Part model, mm, in its own coordinate system. A direction names the side the tool comes from. Round coordinates to 2 decimals unless told otherwise and drop trailing zeros. Write each loop counter-clockwise with the first axis right and the second up, starting at its lowest first coordinate (ties: lowest second). Pieces come first, ordered by that corner, then holes.
1) Which spindle directions (+Z, -Z, +X, -X, +Y, -Y) get a long thin tool onto all of the face, cutting with end or side? Do faces 4 (the flat face through (0, 48, -54)), 5 (the flat face through (-10, 63.4, -58)), 6 (the flat face through (-4, 48, -41)), 7 (the flat face through (41, 48, 4)), 8 (the cylindrical face through (63.85, 64.96, 9.86)). Say none if no direction does.
2) Flat gauge pins, fed straight in: pin 1 (8 mm diameter, centred on x = 19.5, y = 34, fed in from -Z); pin 2 (11 mm diameter, centred on y = 35.5, z = -31.5, fed in from +X); pin 3 (10.5 mm diameter, centred on y = 31.5, z = -55, fed in from +X). Where does each tip first touch, or does it go through?
3) Saw through at C-C on z = -26. Write the cut outline in (x, y).
4) Saw through at D-D on x = 39. Write the cut outline in (y, z).
5) Saw through at A-A on x = -5. Write the cut outline in (y, z).
6) Pull direction Y, two halves, no side cores. Call faces 1 (the flat face through (65.75, 48, 9)), 2 (the flat face through (58, 46.6, 10)), 3 (the cylindrical face through (52.65, 25.04, 9.86)): +Y half, -Y half, draft (parallel to the pull), parting line (faces both ways), or undercut.
7) Saw through at B-B on y = 80.5. Write the cut outline in (x, z), and give its area (3 significant figures).
8) Drill centre lines: L1, parallel to Z at x = 14, y = 57.5; L2, parallel to Z at x = -6, y = 28; L3, parallel to Z at x = 52.5, y = 51. Where is each one in solid material? Low to high.
```python
from build123d import *

# Parameters (mm, degrees)
BOSS_EXTRUDE1_DEPTH = 100
SKETCH2_W           = 37
SKETCH2_H           = 112.688383797
CUT_EXTRUDE1_DEPTH  = 7
SKETCH3_W           = 37
SKETCH3_H           = 114.700676364
CUT_EXTRUDE2_DEPTH  = 7
CUT_EXTRUDE3_DEPTH  = 148.228139294
CUT_EXTRUDE4_DEPTH  = 137.550814717
FILLET1_R           = 10
FILLET2_R           = 2
FILLET3_R           = 2
FILLET4_R           = 2


with BuildPart() as part:
    # Sketch1 → Boss-Extrude1 (new body)
    with BuildSketch(Plane(origin=(0, 0, 0), x_dir=(1, 0, 0), z_dir=(0, 1, 0))):
        Polygon((0, 0), (65.75, 0), (65.75, -20), (-20, -20), (-20, 65.75), (0, 65.75), align=None)
    extrude(amount=BOSS_EXTRUDE1_DEPTH)

    # Sketch2 → Cut-Extrude1 (cut)
    with BuildSketch(Plane(origin=(0, 0, 0), x_dir=(0, 0, -1), z_dir=(1, 0, 0))):
        with Locations((22.5, 52.54890392)):
            Rectangle(SKETCH2_W, SKETCH2_H)
    extrude(amount=-CUT_EXTRUDE1_DEPTH, mode=Mode.SUBTRACT)

    # Sketch3 → Cut-Extrude2 (cut)
    with BuildSketch(Plane(origin=(0, 0, 0), x_dir=(-1, 0, 0), z_dir=(0, 0, -1))):
        with Locations((-22.5, 48.993853716)):
            Rectangle(SKETCH3_W, SKETCH3_H)
    extrude(amount=-CUT_EXTRUDE2_DEPTH, mode=Mode.SUBTRACT)

    # Sketch4 → Cut-Extrude3 (cut, through all)
    with BuildSketch(Plane.ZY.offset(20)):
        with BuildLine():
            Line((-62.25, 86.6), (-54.25, 86.6))
            ThreePointArc((-54.25, 86.6), (-52.65, 85), (-54.25, 83.4))
            Line((-54.25, 83.4), (-62.25, 83.4))
            ThreePointArc((-62.25, 83.4), (-63.85, 85), (-62.25, 86.6))
        make_face()
        with BuildLine():
            Line((-62.25, 66.6), (-54.25, 66.6))
            ThreePointArc((-54.25, 66.6), (-52.65, 65), (-54.25, 63.4))
            Line((-54.25, 63.4), (-62.25, 63.4))
            ThreePointArc((-62.25, 63.4), (-63.85, 65), (-62.25, 66.6))
        make_face()
        with BuildLine():
            Line((-62.25, 46.6), (-54.25, 46.6))
            ThreePointArc((-54.25, 46.6), (-52.65, 45), (-54.25, 43.4))
            Line((-54.25, 43.4), (-62.25, 43.4))
            ThreePointArc((-62.25, 43.4), (-63.85, 45), (-62.25, 46.6))
        make_face()
        with BuildLine():
            Line((-62.25, 26.6), (-54.25, 26.6))
            ThreePointArc((-54.25, 26.6), (-52.65, 25), (-54.25, 23.4))
            Line((-54.25, 23.4), (-62.25, 23.4))
            ThreePointArc((-62.25, 23.4), (-63.85, 25), (-62.25, 26.6))
        make_face()
    extrude(amount=-CUT_EXTRUDE3_DEPTH, mode=Mode.SUBTRACT)

    # Sketch6 → Cut-Extrude4 (cut, through all)
    with BuildSketch(Plane(origin=(0, 0, 0), x_dir=(-1, 0, 0), z_dir=(0, 0, -1))):
        with BuildLine():
            Line((-62.25, 86.6), (-54.25, 86.6))
            ThreePointArc((-54.25, 86.6), (-52.65, 85), (-54.25, 83.4))
            Line((-54.25, 83.4), (-62.25, 83.4))
            ThreePointArc((-62.25, 83.4), (-63.85, 85), (-62.25, 86.6))
        make_face()
        with BuildLine():
            Line((-62.25, 66.6), (-54.25, 66.6))
            ThreePointArc((-54.25, 66.6), (-52.65, 65), (-54.25, 63.4))
            Line((-54.25, 63.4), (-62.25, 63.4))
            ThreePointArc((-62.25, 63.4), (-63.85, 65), (-62.25, 66.6))
        make_face()
        with BuildLine():
            Line((-62.25, 46.6), (-54.25, 46.6))
            ThreePointArc((-54.25, 46.6), (-52.65, 45), (-54.25, 43.4))
            Line((-54.25, 43.4), (-62.25, 43.4))
            ThreePointArc((-62.25, 43.4), (-63.85, 45), (-62.25, 46.6))
        make_face()
        with BuildLine():
            Line((-62.25, 26.6), (-54.25, 26.6))
            ThreePointArc((-54.25, 26.6), (-52.65, 25), (-54.25, 23.4))
            Line((-54.25, 23.4), (-62.25, 23.4))
            ThreePointArc((-62.25, 23.4), (-63.85, 25), (-62.25, 26.6))
        make_face()
    extrude(amount=-CUT_EXTRUDE4_DEPTH, mode=Mode.SUBTRACT)

    # Fillet1
    fillet1_edges = [part.edges().sort_by_distance(p)[0] for p in [
        (-20, 50, 20),
    ]]
    fillet(fillet1_edges, radius=FILLET1_R)

    # Fillet2
    fillet2_edges = [part.edges().sort_by_distance(p)[0] for p in [
        (0, 50, -41),
        (0, 50, -4),
        (4, 50, 0),
        (41, 50, 0),
    ]]
    fillet(fillet2_edges, radius=FILLET2_R)

    # Fillet3
    fillet3_edges = [part.edges().sort_by_distance(p)[0] for p in [
        (-20, 100, -27.875),
        (65.75, 100, 10),
        (27.875, 100, 20),
        (-17.071067812, 100, 17.071067812),
        (4, 100, 4.5),
        (1, 100, 0),
        (-4.5, 100, -41),
        (0, 100, -54.375),
        (-0.585786438, 100, -3.414213562),
        (-0.585786438, 100, -41.585786438),
        (3.414213562, 100, 0.585786438),
        (41.585786438, 100, 0.585786438),
        (54.375, 100, 0),
        (-4.5, 100, -4),
        (-7, 100, -22.5),
        (0, 100, -1),
        (41, 100, 4.5),
        (22.5, 100, 7),
        (-10, 100, -65.75),
    ]]
    fillet(fillet3_edges, radius=FILLET3_R)

    # Fillet4
    # the kernel refuses this fillet: 2 mm, written as the material it takes off along each edge
    with BuildSketch(Plane(origin=(-2, 98, -63.75), x_dir=(0, 0, -1), z_dir=(1, 0, 0))) as fillet4_piece_1_section:
        Polygon((0, 0), (FILLET4_R, 0), (FILLET4_R, FILLET4_R), (0, FILLET4_R), align=None)
    fillet4_piece_1 = extrude(amount=FILLET4_R, mode=Mode.PRIVATE)
    fillet4_piece_1 = fillet4_piece_1 - Plane(origin=(-2, 98, -63.75), x_dir=(0, -0.7071067811865475, 0.7071067811865475), z_dir=(1, 0, 0)) * Sphere(FILLET4_R, mode=Mode.PRIVATE)
    add(fillet4_piece_1, mode=Mode.SUBTRACT)
    with BuildSketch(Plane(origin=(63.75, 98, 18), x_dir=(1, 0, 0), z_dir=(0, 0, 1))) as fillet4_piece_2_section:
        Polygon((0, 0), (FILLET4_R, 0), (FILLET4_R, FILLET4_R), (0, FILLET4_R), align=None)
    fillet4_piece_2 = extrude(amount=FILLET4_R, mode=Mode.PRIVATE)
    fillet4_piece_2 = fillet4_piece_2 - Plane(origin=(63.75, 98, 18), x_dir=(-0.7071067811865475, -0.7071067811865475, 0), z_dir=(0, 0, 1)) * Sphere(FILLET4_R, mode=Mode.PRIVATE)
    add(fillet4_piece_2, mode=Mode.SUBTRACT)
    with BuildSketch(Plane(origin=(65.75, -5, 20), x_dir=(-1, 0, 0), z_dir=(0, 1, 0)), Plane(origin=(0, -5, -65.75), x_dir=(0, 0, 1), z_dir=(0, 1, 0))) as fillet4_piece_3:
        with BuildLine():
            CenterArc((FILLET4_R, -FILLET4_R), FILLET4_R, 90, 90)
            Line((0, -FILLET4_R), (0, 0))
            Line((0, 0), (FILLET4_R, 0))
        make_face()
    extrude(amount=103, mode=Mode.SUBTRACT)


solid = part.part
```
Completed:
1. face 4: -Z, +X, +Y, -Y
1. face 5: +X, -X
1. face 6: +X, +Y, -Y
1. face 7: -Z, +Y, -Y
1. face 8: +Z, -Z
2. pin 1: stops at z = 7
2. pin 2: stops at x = -7
2. pin 3: stops at x = 0
3. outline: (-20, 0) - (-7, 0) - (-7, 98) arc R2 ccw to (-9, 100) - (-18, 100) arc R2 ccw to (-20, 98) - close
4. outline: (0, 7) - (98, 7) arc R2 ccw to (100, 9) - (100, 18) arc R2 ccw to (98, 20) - (0, 20) - close
5. outline: (0, -65.75) - (98, -65.75) arc R2 ccw to (100, -63.75) - (100, -43) arc R2 ccw to (98, -41) - (0, -41) - close; (0, -4) - (98, -4) arc R2 ccw to (100, -2) - (100, 18) arc R2 ccw to (98, 20) - (0, 20) - close; hole (23.4, -62.25) arc R1.6 ccw to (26.6, -62.25) - (26.6, -54.25) arc R1.6 ccw to (23.4, -54.25) - close; hole (43.4, -62.25) arc R1.6 ccw to (46.6, -62.25) - (46.6, -54.25) arc R1.6 ccw to (43.4, -54.25) - close; hole (63.4, -62.25) arc R1.6 ccw to (66.6, -62.25) - (66.6, -54.25) arc R1.6 ccw to (63.4, -54.25) - close; hole (83.4, -62.25) arc R1.6 ccw to (86.6, -62.25) - (86.6, -54.25) arc R1.6 ccw to (83.4, -54.25) - close
6. face 1: draft
6. face 2: undercut
6. face 3: undercut
7. outline: (-20, -65.75) - (-2, -65.75) arc R2 ccw to (0, -63.75) - (0, -43) arc R2 ccw to (-2, -41) - (-7, -41) - (-7, -4) - (-2, -4) arc R2 ccw to (0, -2) - (0, 0) - (2, 0) arc R2 ccw to (4, 2) - (4, 7) - (41, 7) - (41, 2) arc R2 ccw to (43, 0) - (65.75, 0) - (65.75, 18) arc R2 ccw to (63.75, 20) - (-10, 20) arc R10 ccw to (-20, 10) - close
7. area: 2,490 mm2
8. L1: z = 7 to 20
8. L2: z = -65.75 to -41, -4 to 20
8. L3: z = 0 to 20
